from build123d import *

# Parameters (mm, degrees)
SKETCH1_2_W         = 400
SKETCH1_2_H         = 285
SKETCH1_2_W_2       = 20
SKETCH1_2_H_2       = 5
SKETCH1_2_W_3       = 5
SKETCH1_2_H_3       = 20
BOSS_EXTRUDE3_DEPTH = 2.5
FILLET2_R           = 5


with BuildPart() as part:
    # Sketch1<2> → Boss-Extrude3 (new body)
    with BuildSketch(Plane(origin=(0, 0, 0), x_dir=(0, 0, -1), z_dir=(1, 0, 0))):
        Rectangle(SKETCH1_2_W, SKETCH1_2_H)
        with Locations((-170, 135)):
            Rectangle(SKETCH1_2_W_2, SKETCH1_2_H_2, mode=Mode.SUBTRACT)
        with Locations((-170, -135)):
            Rectangle(SKETCH1_2_W_2, SKETCH1_2_H_2, mode=Mode.SUBTRACT)
        with Locations((-127.5, 135)):
            Rectangle(SKETCH1_2_W_2, SKETCH1_2_H_2, mode=Mode.SUBTRACT)
        with Locations((-127.5, -135)):
            Rectangle(SKETCH1_2_W_2, SKETCH1_2_H_2, mode=Mode.SUBTRACT)
        with Locations((-85, 135)):
            Rectangle(SKETCH1_2_W_2, SKETCH1_2_H_2, mode=Mode.SUBTRACT)
        with Locations((-85, -135)):
            Rectangle(SKETCH1_2_W_2, SKETCH1_2_H_2, mode=Mode.SUBTRACT)
        with Locations((-42.5, 135)):
            Rectangle(SKETCH1_2_W_2, SKETCH1_2_H_2, mode=Mode.SUBTRACT)
        with Locations((-42.5, -135)):
            Rectangle(SKETCH1_2_W_2, SKETCH1_2_H_2, mode=Mode.SUBTRACT)
        with Locations((0, 135)):
            Rectangle(SKETCH1_2_W_2, SKETCH1_2_H_2, mode=Mode.SUBTRACT)
        with Locations((0, -135)):
            Rectangle(SKETCH1_2_W_2, SKETCH1_2_H_2, mode=Mode.SUBTRACT)
        with Locations((42.5, 135)):
            Rectangle(SKETCH1_2_W_2, SKETCH1_2_H_2, mode=Mode.SUBTRACT)
        with Locations((42.5, -135)):
            Rectangle(SKETCH1_2_W_2, SKETCH1_2_H_2, mode=Mode.SUBTRACT)
        with Locations((85, 135)):
            Rectangle(SKETCH1_2_W_2, SKETCH1_2_H_2, mode=Mode.SUBTRACT)
        with Locations((85, -135)):
            Rectangle(SKETCH1_2_W_2, SKETCH1_2_H_2, mode=Mode.SUBTRACT)
        with Locations((127.5, 135)):
            Rectangle(SKETCH1_2_W_2, SKETCH1_2_H_2, mode=Mode.SUBTRACT)
        with Locations((127.5, -135)):
            Rectangle(SKETCH1_2_W_2, SKETCH1_2_H_2, mode=Mode.SUBTRACT)
        with Locations((170, 135)):
            Rectangle(SKETCH1_2_W_2, SKETCH1_2_H_2, mode=Mode.SUBTRACT)
        with Locations((170, -135)):
            Rectangle(SKETCH1_2_W_2, SKETCH1_2_H_2, mode=Mode.SUBTRACT)
        with Locations((192.5, 112.5)):
            Rectangle(SKETCH1_2_W_3, SKETCH1_2_H_3, mode=Mode.SUBTRACT)
        with Locations((-192.5, 112.5)):
            Rectangle(SKETCH1_2_W_3, SKETCH1_2_H_3, mode=Mode.SUBTRACT)
        with Locations((-192.5, 67.5)):
            Rectangle(SKETCH1_2_W_3, SKETCH1_2_H_3, mode=Mode.SUBTRACT)
        with Locations((192.5, 67.5)):
            Rectangle(SKETCH1_2_W_3, SKETCH1_2_H_3, mode=Mode.SUBTRACT)
        with Locations((-192.5, 22.5)):
            Rectangle(SKETCH1_2_W_3, SKETCH1_2_H_3, mode=Mode.SUBTRACT)
        with Locations((192.5, 22.5)):
            Rectangle(SKETCH1_2_W_3, SKETCH1_2_H_3, mode=Mode.SUBTRACT)
        with Locations((-192.5, -22.5)):
            Rectangle(SKETCH1_2_W_3, SKETCH1_2_H_3, mode=Mode.SUBTRACT)
        with Locations((192.5, -22.5)):
            Rectangle(SKETCH1_2_W_3, SKETCH1_2_H_3, mode=Mode.SUBTRACT)
        with Locations((-192.5, -67.5)):
            Rectangle(SKETCH1_2_W_3, SKETCH1_2_H_3, mode=Mode.SUBTRACT)
        with Locations((192.5, -67.5)):
            Rectangle(SKETCH1_2_W_3, SKETCH1_2_H_3, mode=Mode.SUBTRACT)
        with Locations((-192.5, -112.5)):
            Rectangle(SKETCH1_2_W_3, SKETCH1_2_H_3, mode=Mode.SUBTRACT)
        with Locations((192.5, -112.5)):
            Rectangle(SKETCH1_2_W_3, SKETCH1_2_H_3, mode=Mode.SUBTRACT)
    extrude(amount=BOSS_EXTRUDE3_DEPTH)

    # Fillet2
    fillet2_edges = [part.edges().sort_by_distance(p)[0] for p in [
        (1.25, -142.5, 200),
        (1.25, 142.5, 200),
        (1.25, 142.5, -200),
        (1.25, -142.5, -200),
    ]]
    fillet(fillet2_edges, radius=FILLET2_R)


solid = part.part
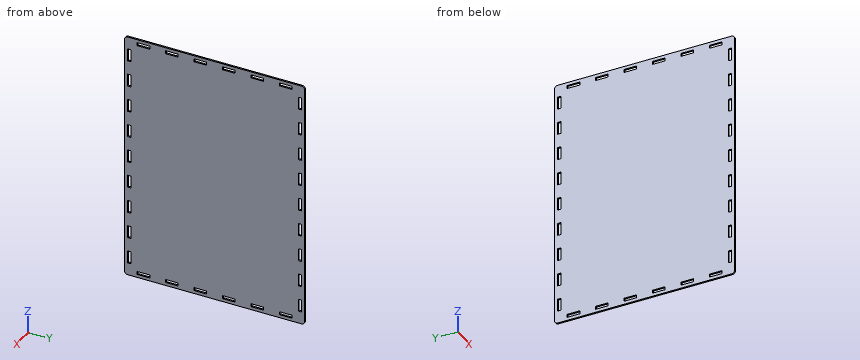
The model under review builds one solid part; all positions refer to its coordinate system, in mm. Coordinates: 2 decimals unless noted, no trailing zeros. Order: outer loops, then holes, each group sorted by start corner. A loop starts at its lowest first (then second) coordinate and runs counter-clockwise, first axis right, second up. Notation, with made-up numbers: (75, 83.25) -> (104, 83.25) arc R29 cw to (104, 120.25) -> close; hole circle Ø8 at (49, -36). An arc over 180 degrees is marked (long way). Answer in a Markdown table with one row per item.
(1) Consider section B-B (y = 110). Write out the cut boundary in (x, z), plus the area to 3 significant figures.
Answers:
| item | result |
|---|---|
| outline | (0, -200) -> (2.5, -200) -> (2.5, -195) -> (0, -195) -> close; (0, -190) -> (2.5, -190) -> (2.5, 190) -> (0, 190) -> close; (0, 195) -> (2.5, 195) -> (2.5, 200) -> (0, 200) -> close |
| area | 975 mm² |
(2) Consider section A-A (z = 132.5). Write out the cut boundary in (x, y), plus the area to 4 significant figures.
Answers:
| item | result |
|---|---|
| outline | (0, -142.5) -> (2.5, -142.5) -> (2.5, -137.5) -> (0, -137.5) -> close; (0, -132.5) -> (2.5, -132.5) -> (2.5, 132.5) -> (0, 132.5) -> close; (0, 137.5) -> (2.5, 137.5) -> (2.5, 142.5) -> (0, 142.5) -> close |
| area | 687.5 mm² |
(3) Consider section C-C (x = 0.45). State how many separate pieces and enclosed holes the cut face has, plus the area to 3 significant figures.
Answers:
| item | result |
|---|---|
| separate pieces | 1 |
| enclosed holes | 30 |
| area | 111,000 mm² |
(4) Wall thickness on line 1 along Y through (x, z) = (2, 126); line 2 along Z through (x, y) = (1.4, -117): over which ranges is each line inside the solid? List them lowest first.
Answers:
| item | result |
|---|---|
| line 1 | -142.5 to -137.5, -132.5 to 132.5, 137.5 to 142.5 |
| line 2 | -200 to -195, -190 to 190, 195 to 200 |
